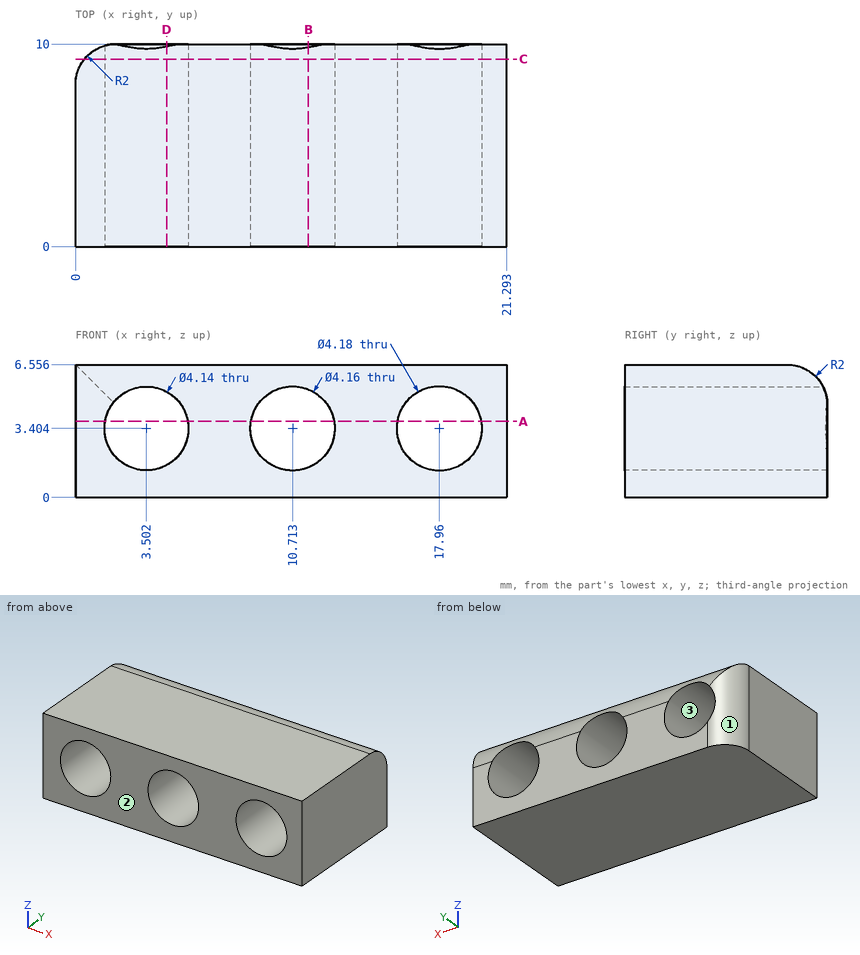
Check sheet for the drawn part. Datum: minimum x, y, z corner. Units: mm. Round coordinates to 2 decimals unless told otherwise and drop trailing zeros. Write each loop counter-clockwise with the first axis right and the second up, starting at its lowest first coordinate (ties: lowest second). Pieces come first, ordered by that corner, then holes. Notation, with made-up numbers: (9, 70.25) - (24, 70.25) arc R26 cw to (24, 89.25) - close; hole circle Ø11 at (-2, -24). An arc over 180 degrees is marked (long way). Write each question's results on one line, items separated by ' | '.
(1) Sectioned sample at D-D, the plane x = 4.5. Enter the section's corners in (y, z).
Computed:
outline: (0, 0) - (10, 0) - (10, 1.59) - (0, 1.59) - close; (0, 5.22) - (9.89, 5.22) arc R2 ccw to (8, 6.56) - (0, 6.56) - close
(2) Draft check along X on the marked faces 1, 2 and 3. Enter one of: pulls with the +X half, pulls with the -X half, needs draft (parallel to the pull), parting line crosses it, or undercut.
Computed:
face 1: pulls with the -X half | face 2: needs draft | face 3: undercut
(3) Thickness scan on probe 1 along X at (y, z) = (5.5, 4) (1 decimal); probe 2 along X at (y, z) = (8.25, 2.25) (1 decimal); probe 3 along Z at (x, y) = (18.25, 6.5) (1 decimal). Record the ranges inside material, lowest first. Write a range as from..to.
Computed:
probe 1: x = 0..1.5, 5.5..8.7, 12.7..16, 20..21.3 | probe 2: x = 0..1.8, 5.2..9, 12.4..16.2, 19.7..21.3 | probe 3: z = 0..1.3, 5.5..6.6
(4) Sectioned sample at B-B, the plane x = 11.5. Enter the section's corners in (y, z) (1 decimal).
Computed:
outline: (0, 0) - (10, 0) - (10, 1.5) - (0, 1.5) - close; (0, 5.3) - (9.8, 5.3) arc R2 ccw to (8, 6.6) - (0, 6.6) - close
(5) Sectioned sample at A-A, the plane z = 3.75. Enter the section's corners in (x, y).
Computed:
outline: (0, 0) - (1.46, 0) - (1.46, 9.93) arc R2 ccw to (0, 8) - close; (5.54, 0) - (8.66, 0) - (8.66, 10) - (5.54, 10) - close; (12.76, 0) - (15.9, 0) - (15.9, 10) - (12.76, 10) - close; (20.02, 0) - (21.29, 0) - (21.29, 10) - (20.02, 10) - close
(6) Sectioned sample at C-C, the plane y = 9.25. Enter the section's corners in (x, z) (1 decimal).
Computed:
outline: (0.4, 0) - (21.3, 0) - (21.3, 6.1) - (0.4, 6.1) - close; hole circle Ø4.1 at (3.5, 3.4); hole circle Ø4.2 at (10.7, 3.4); hole circle Ø4.2 at (18, 3.4)
